Part model, mm, in its own coordinate system. Face numbers are marked on the shaded views. Round coordinates to 2 decimals unless told otherwise and drop trailing zeros. Write each loop counter-clockwise with the first axis right and the second up, starting at its lowest first coordinate (ties: lowest second). Pieces come first, ordered by that corner, then holes.
1) Flat gauge pins, fed straight in: pin 1 (12 mm diameter, centred on x = -39, z = 14, fed in from -Y); pin 2 (6 mm diameter, centred on x = -21.5, z = 3, fed in from +Y); pin 3 (3 mm diameter, centred on x = -12.7, z = 12.7, fed in from +Y). Where does each tip first touch, or does it go through?
2) Drill centre lines: L1, parallel to Z at x = -1, y = 38; L2, parallel to Y at x = -0.9, z = 12.7; L3, parallel to Y at x = -1.75, z = 12.7. Where is each one in solid material? Low to high.
3) Saw through at C-C on x = -12.7. Write the cut outline in (y, z), and give its area (3 significant figures).
4) Saw through at A-A on y = 38.1. Write the cut outline in (x, z), and give its area (3 significant figures).
5) Saw through at D-D on y = 107. Write the cut outline in (x, z), and give its area (3 significant figures).
6) Saw through at B-B on z = 12.7. Write the cut outline in (x, y), and give its area (3 significant figures).
7) Pull direction Y, two halves, no side cores. Call the marked faces 1, 2 and 3: +Y half, -Y half, draft (parallel to the pull), parting line (faces both ways), or undercut.
```python
from build123d import *

# Parameters (mm, degrees)
BASE_FLANGE1_DEPTH = 25.4
CUT_EXTRUDE1_REACH = 253.219
SKETCH3_R          = 2.7051
CUT_EXTRUDE2_REACH = 220.156
SKETCH4_R          = 2.7051
CUT_EXTRUDE3_REACH = 253.219
SKETCH5_R          = 2.7051


# Sheet-metal steps are written as plain solids
with BuildPart() as part:
    # Sketch1 → Base-Flange1 (new body)
    with BuildSketch(Plane.XY):
        with BuildLine():
            Line((-25.4, 0), (-4.0132, 0))
            ThreePointArc((-4.0132, 0), (-1.175439066, 1.175439066), (0, 4.0132))
            Line((0, 4.0132), (0, 176.137678131))
            ThreePointArc((0, 176.137678131), (-0.30548666, 177.673463282), (-1.175439066, 178.975439066))
            Line((-1.175439066, 178.975439066), (-63.5, 241.3))
            Line((-63.5, 241.3), (-65.116446102, 239.683553898))
            Line((-65.116446102, 239.683553898), (-2.791885168, 177.358992964))
            ThreePointArc((-2.791885168, 177.358992964), (-2.417475271, 176.798648956), (-2.286, 176.137678131))
            Line((-2.286, 176.137678131), (-2.286, 4.0132))
            ThreePointArc((-2.286, 4.0132), (-2.791885168, 2.791885168), (-4.0132, 2.286))
            Line((-4.0132, 2.286), (-25.4, 2.286))
            Line((-25.4, 2.286), (-25.4, 0))
        make_face()
    extrude(amount=BASE_FLANGE1_DEPTH)

    # Sketch3 → Cut-Extrude1 (cut, up to next)
    with BuildSketch(Plane(origin=(0, 0, 0), x_dir=(0, 0, -1), z_dir=(1, 0, 0)), mode=Mode.PRIVATE) as cut_extrude1_sk1:
        with Locations((-12.7, 38.1)):
            Circle(SKETCH3_R)
    cut_extrude1_tool1 = extrude(cut_extrude1_sk1.sketch, amount=-CUT_EXTRUDE1_REACH, mode=Mode.PRIVATE) & part.part
    # Sketch3 → Cut-Extrude1 (cut, up to next)
    with BuildSketch(Plane(origin=(0, 0, 0), x_dir=(0, 0, -1), z_dir=(1, 0, 0)), mode=Mode.PRIVATE) as cut_extrude1_sk2:
        with Locations((-12.7, 139.7)):
            Circle(SKETCH3_R)
    cut_extrude1_tool2 = extrude(cut_extrude1_sk2.sketch, amount=-CUT_EXTRUDE1_REACH, mode=Mode.PRIVATE) & part.part
    add(cut_extrude1_tool1.solids().sort_by_distance((0, 38.1, 12.7))[0], mode=Mode.SUBTRACT)
    add(cut_extrude1_tool2.solids().sort_by_distance((0, 139.7, 12.7))[0], mode=Mode.SUBTRACT)

    # Sketch4 → Cut-Extrude2 (cut, up to next)
    with BuildSketch(Plane(origin=(88.9, 88.9, 0), x_dir=(0, 0, -1), z_dir=(0.7071067811865462, 0.7071067811865489, 0)), mode=Mode.PRIVATE) as cut_extrude2_sk1:
        with Locations(Location((-12.7, 176.523585695, 0), (0, 0, 90))):
            Circle(SKETCH4_R)
    cut_extrude2_tool1 = extrude(cut_extrude2_sk1.sketch, amount=-CUT_EXTRUDE2_REACH, mode=Mode.PRIVATE) & part.part
    add(cut_extrude2_tool1.solids().sort_by_distance((-35.921024, 213.721024, 12.7))[0], mode=Mode.SUBTRACT)

    # Sketch5 → Cut-Extrude3 (cut, up to next)
    with BuildSketch(Plane.XZ, mode=Mode.PRIVATE) as cut_extrude3_sk1:
        with Locations((-12.7, 12.7)):
            Circle(SKETCH5_R)
    cut_extrude3_tool1 = extrude(cut_extrude3_sk1.sketch, amount=-CUT_EXTRUDE3_REACH, mode=Mode.PRIVATE) & part.part
    add(cut_extrude3_tool1.solids().sort_by_distance((-12.7, 0, 12.7))[0], mode=Mode.SUBTRACT)


solid = part.part
```
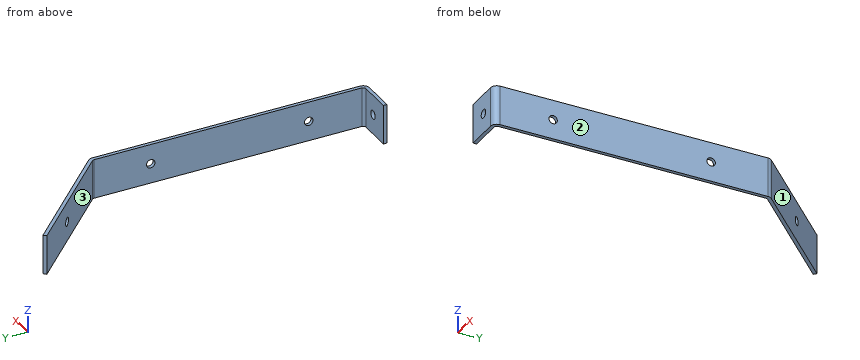
Completed:
1. pin 1: stops at y = 207.57
1. pin 2: stops at y = 202.3
1. pin 3: stops at y = 192
2. L1: z = 0 to 10, 15.4 to 25.4
2. L2: y = 1.48 to 35.39, 40.81 to 136.99, 142.41 to 178.67
2. L3: y = 0.7 to 35.39, 40.81 to 136.99, 142.41 to 179.55
3. outline: (0, 0) - (2.29, 0) - (2.29, 9.99) - (0, 9.99) - close; (0, 15.41) - (2.29, 15.41) - (2.29, 25.4) - (0, 25.4) - close; (187.27, 0) - (190.5, 0) - (190.5, 25.4) - (187.27, 25.4) - close
3. area: 128 mm2
4. outline: (-2.29, 0) - (0, 0) - (0, 9.99) - (-2.29, 9.99) - close; (-2.29, 15.41) - (0, 15.41) - (0, 25.4) - (-2.29, 25.4) - close
4. area: 45.7 mm2
5. outline: (-2.29, 0) - (0, 0) - (0, 25.4) - (-2.29, 25.4) - close
5. area: 58.1 mm2
6. outline: (-65.12, 239.68) - (-39.45, 214.02) - (-37.83, 215.63) - (-63.5, 241.3) - close; (-35.62, 210.19) - (-2.79, 177.36) arc R1.73 cw to (-2.29, 176.14) - (-2.29, 142.41) - (0, 142.41) - (0, 176.14) arc R4.01 ccw to (-1.18, 178.98) - (-34.01, 211.81) - close; (-25.4, 0) - (-15.41, 0) - (-15.41, 2.29) - (-25.4, 2.29) - close; (-9.99, 0) - (-4.01, 0) arc R4.01 ccw to (0, 4.01) - (0, 35.39) - (-2.29, 35.39) - (-2.29, 4.01) arc R1.73 cw to (-4.01, 2.29) - (-9.99, 2.29) - close; (-2.29, 40.81) - (0, 40.81) - (0, 136.99) - (-2.29, 136.99) - close
6. area: 610 mm2
7. face 1: +Y half
7. face 2: draft
7. face 3: undercut
